For this review, take the finished solid that the model builds, in its own axes (mm). A direction names the side the tool comes from. Coordinates: 2 decimals unless noted, no trailing zeros. Write each loop counter-clockwise with the first axis right and the second up, starting at its lowest first coordinate (ties: lowest second). Pieces come first, ordered by that corner, then holes. Notation, with made-up numbers: (-37, -3.5) - (-13, -3.5) arc R34 cw to (-13, 28.5) - close; hole circle Ø5 at (57.5, 20). An arc over 180 degrees is marked (long way). Use one line per item in the form item = value. Start each with the question number.
1) Mouldability with a two-part tool opening along Z and no side actions: class faces 4 (the flat face through (-12, 0, -1)), 5 (the flat face through (-2, 5, 37)) as pulls with the +Z half, pulls with the -Z half, needs draft (parallel to the pull), parting line crosses it, or undercut.
2) We need section C-C (x = -50). Give the boundary of the cut face in (y, z).
3) We need section D-D (z = 50.5). Give the boundary of the cut face in (x, y), plus the area to 3 significant figures.
4) Tool access review of faces 1 (the cylindrical face through (-34.94, 8.45, 12.73)), 2 (the cylindrical face through (14.898, 2.465, 39.316)), 3 (the cylindrical face through (-5.41, 4.51, 5.34)): name each direction out of +Z, -Z, +X, -X, +Y, -Y from which nothing blocks a thin tool from reaching the whole face with its end or side.
5) We need section B-B (x = -20). Give the boundary of the cut face in (y, z), plus the area to 3 significant figures.
6) For L1, parallel to X at y = 11.75, z = -14; L2, parallel to Z at x = 16, y = 9; L3, parallel to X at y = 6.75, z = 27.5, list the stretches that pass through material, from the lowest coordinate up. Write a range as from..to.
7) We need section A-A (z = -20). Give the boundary of the cut face in (x, y), plus the area to 3 significant figures.
8) Insertion check: P1, Ø12, axis at y = 17, z = -36, coming from the -X side; P2, Ø2, axis at x = -10, y = 4.5, coming from the +Z side; P3, Ø8, axis at x = -17, y = 7.5, coming from the +Z side. Each pin has a flat end and moves straight along its axis. Give the tip position at first contact, or say it passes through.
```python
from build123d import *

# Parameters (mm, degrees)
SKETCH_1_R           = 59
EXTRUDE_1_DEPTH      = 20
SKETCH_2_R           = 44.5
CUT_EXTRUDE_1_DEPTH  = 8
SKETCH_3_R           = 30.1
CUT_EXTRUDE_2_DEPTH  = 6.5
SKETCH_4_R           = 2.1
CUT_EXTRUDE_3_DEPTH  = 86.802097876
SKETCH_5_R           = 3.75
CUT_EXTRUDE_4_DEPTH  = 5
M6X1_0_2_D           = 5
SKETCH_26_R          = 3.1
CUT_EXTRUDE_14_DEPTH = 1.2
CUT_EXTRUDE_17_DEPTH = 2
FILLET_1_R           = 1
SKETCH_29_R          = 1.6
CUT_EXTRUDE_18_DEPTH = 86.530345492


with BuildPart() as part:
    # 草图1 → 凸台-拉伸1 (new body)
    with BuildSketch(Plane(origin=(0, 0, 0), x_dir=(1, 0, 0), z_dir=(0, 1, 0))):
        with Locations(Location((0, 0, 0), (0, 0, 270))):
            Circle(SKETCH_1_R)
    extrude(amount=EXTRUDE_1_DEPTH)

    # 草图2 → 切除-拉伸1 (cut)
    with BuildSketch(Plane(origin=(0, 20, 0), x_dir=(1, 0, 0), z_dir=(0, 1, 0))):
        with Locations(Location((0, 0, 0), (0, 0, 270))):
            Circle(SKETCH_2_R)
    extrude(amount=-CUT_EXTRUDE_1_DEPTH, mode=Mode.SUBTRACT)

    # 草图3 → 切除-拉伸2 (cut)
    with BuildSketch(Plane(origin=(0, 12, 0), x_dir=(1, 0, 0), z_dir=(0, 1, 0))):
        with Locations(Location((0, 0, 0), (0, 0, 270))):
            Circle(SKETCH_3_R)
    extrude(amount=-CUT_EXTRUDE_2_DEPTH, mode=Mode.SUBTRACT)

    # 草图4 → 切除-拉伸3 (cut, through all)
    with BuildSketch(Plane.XZ):
        with Locations(Location((0, 38.5, 0), (0, 0, 270))):
            Circle(SKETCH_4_R)
        with Locations(Location((14.733312146, 35.569362002, 0), (0, 0, 270))):
            Circle(SKETCH_4_R)
        with Locations(Location((27.223611076, 27.223611076, 0), (0, 0, 270))):
            Circle(SKETCH_4_R)
        with Locations(Location((35.569362002, 14.733312146, 0), (0, 0, 270))):
            Circle(SKETCH_4_R)
        with Locations(Location((38.5, 0, 0), (0, 0, 270))):
            Circle(SKETCH_4_R)
        with Locations(Location((35.569362002, -14.733312146, 0), (0, 0, 270))):
            Circle(SKETCH_4_R)
        with Locations(Location((27.223611076, -27.223611076, 0), (0, 0, 270))):
            Circle(SKETCH_4_R)
        with Locations(Location((14.733312146, -35.569362002, 0), (0, 0, 270))):
            Circle(SKETCH_4_R)
        with Locations(Location((0, -38.5, 0), (0, 0, 270))):
            Circle(SKETCH_4_R)
        with Locations(Location((-14.733312146, -35.569362002, 0), (0, 0, 270))):
            Circle(SKETCH_4_R)
        with Locations(Location((-27.223611076, -27.223611076, 0), (0, 0, 270))):
            Circle(SKETCH_4_R)
        with Locations(Location((-35.569362002, -14.733312146, 0), (0, 0, 270))):
            Circle(SKETCH_4_R)
        with Locations(Location((-38.5, 0, 0), (0, 0, 270))):
            Circle(SKETCH_4_R)
        with Locations(Location((-35.569362002, 14.733312146, 0), (0, 0, 270))):
            Circle(SKETCH_4_R)
        with Locations(Location((-27.223611076, 27.223611076, 0), (0, 0, 270))):
            Circle(SKETCH_4_R)
        with Locations(Location((-14.733312146, 35.569362002, 0), (0, 0, 270))):
            Circle(SKETCH_4_R)
    extrude(amount=-CUT_EXTRUDE_3_DEPTH, mode=Mode.SUBTRACT)

    # 草图5 → 切除-拉伸4 (cut)
    with BuildSketch(Plane.XZ):
        with Locations(Location((0, 38.5, 0), (0, 0, 270))):
            Circle(SKETCH_5_R)
        with Locations(Location((14.733312146, 35.569362002, 0), (0, 0, 270))):
            Circle(SKETCH_5_R)
        with Locations(Location((27.223611076, 27.223611076, 0), (0, 0, 270))):
            Circle(SKETCH_5_R)
        with Locations(Location((35.569362002, 14.733312146, 0), (0, 0, 270))):
            Circle(SKETCH_5_R)
        with Locations(Location((38.5, 0, 0), (0, 0, 270))):
            Circle(SKETCH_5_R)
        with Locations(Location((35.569362002, -14.733312146, 0), (0, 0, 270))):
            Circle(SKETCH_5_R)
        with Locations(Location((27.223611076, -27.223611076, 0), (0, 0, 270))):
            Circle(SKETCH_5_R)
        with Locations(Location((14.733312146, -35.569362002, 0), (0, 0, 270))):
            Circle(SKETCH_5_R)
        with Locations(Location((0, -38.5, 0), (0, 0, 270))):
            Circle(SKETCH_5_R)
        with Locations(Location((-14.733312146, -35.569362002, 0), (0, 0, 270))):
            Circle(SKETCH_5_R)
        with Locations(Location((-27.223611076, -27.223611076, 0), (0, 0, 270))):
            Circle(SKETCH_5_R)
        with Locations(Location((-35.569362002, -14.733312146, 0), (0, 0, 270))):
            Circle(SKETCH_5_R)
        with Locations(Location((-38.5, 0, 0), (0, 0, 270))):
            Circle(SKETCH_5_R)
        with Locations(Location((-35.569362002, 14.733312146, 0), (0, 0, 270))):
            Circle(SKETCH_5_R)
        with Locations(Location((-27.223611076, 27.223611076, 0), (0, 0, 270))):
            Circle(SKETCH_5_R)
        with Locations(Location((-14.733312146, 35.569362002, 0), (0, 0, 270))):
            Circle(SKETCH_5_R)
    extrude(amount=-CUT_EXTRUDE_4_DEPTH, mode=Mode.SUBTRACT)

    # M6x1.0 螺纹孔2 (through all)
    with Locations(Plane(origin=(0, 0, 0), x_dir=(-1, 0, 0), z_dir=(0, -1, 0))):
        with Locations((0, 20), (-20, 0), (0, -20), (20, 0)):
            Hole(M6X1_0_2_D / 2)

    # 草图26 → 切除-拉伸14 (cut)
    with BuildSketch(Plane.XZ):
        with Locations(Location((0, 0, 0), (0, 0, 270))):
            Circle(SKETCH_26_R)
    extrude(amount=-CUT_EXTRUDE_14_DEPTH, mode=Mode.SUBTRACT)

    # 草图28 → 切除-拉伸17 (cut)
    with BuildSketch(Plane(origin=(0, 5.5, 0), x_dir=(1, 0, 0), z_dir=(0, 1, 0))):
        with BuildLine():
            Line((-2.1, 11), (-2.1, 7.304108433))
            ThreePointArc((-2.1, 7.304108433), (0, 7.6), (2.1, 7.304108433))
            Line((2.1, 7.304108433), (2.1, 11))
            ThreePointArc((2.1, 11), (0, 13.1), (-2.1, 11))
        make_face()
        with BuildLine():
            ThreePointArc((2.1, 5), (0, 2.9), (-2.1, 5))
            Line((-2.1, 5), (-2.1, 7.304108433))
            ThreePointArc((-2.1, 7.304108433), (-5.374011537, 5.374011537), (-7.304108433, 2.1))
            Line((-7.304108433, 2.1), (-5, 2.1))
            ThreePointArc((-5, 2.1), (-2.9, 0), (-5, -2.1))
            Line((-5, -2.1), (-7.304108433, -2.1))
            ThreePointArc((-7.304108433, -2.1), (-5.374011537, -5.374011537), (-2.1, -7.304108433))
            Line((-2.1, -7.304108433), (-2.1, -5))
            ThreePointArc((-2.1, -5), (0, -2.9), (2.1, -5))
            Line((2.1, -5), (2.1, -7.304108433))
            ThreePointArc((2.1, -7.304108433), (5.374011537, -5.374011537), (7.304108433, -2.1))
            Line((7.304108433, -2.1), (5, -2.1))
            ThreePointArc((5, -2.1), (2.9, 0), (5, 2.1))
            Line((5, 2.1), (7.304108433, 2.1))
            ThreePointArc((7.304108433, 2.1), (5.374011537, 5.374011537), (2.1, 7.304108433))
            Line((2.1, 7.304108433), (2.1, 5))
        make_face()
        with BuildLine():
            ThreePointArc((-7.304108433, -2.1), (-7.6, 0), (-7.304108433, 2.1))
            Line((-7.304108433, 2.1), (-11, 2.1))
            ThreePointArc((-11, 2.1), (-13.1, 0), (-11, -2.1))
            Line((-11, -2.1), (-7.304108433, -2.1))
        make_face()
        with BuildLine():
            ThreePointArc((2.1, -7.304108433), (0, -7.6), (-2.1, -7.304108433))
            Line((-2.1, -7.304108433), (-2.1, -11))
            ThreePointArc((-2.1, -11), (0, -13.1), (2.1, -11))
            Line((2.1, -11), (2.1, -7.304108433))
        make_face()
        with BuildLine():
            Line((11, 2.1), (7.304108433, 2.1))
            ThreePointArc((7.304108433, 2.1), (7.525663562, 1.060371612), (7.6, 0))
            ThreePointArc((7.6, 0), (7.525663562, -1.060371612), (7.304108433, -2.1))
            Line((7.304108433, -2.1), (11, -2.1))
            ThreePointArc((11, -2.1), (13.1, 0), (11, 2.1))
        make_face()
        with BuildLine():
            Line((-2.1, 7.304108433), (-2.1, 5))
            ThreePointArc((-2.1, 5), (0, 2.9), (2.1, 5))
            Line((2.1, 5), (2.1, 7.304108433))
            ThreePointArc((2.1, 7.304108433), (0, 7.6), (-2.1, 7.304108433))
        make_face()
        with BuildLine():
            Line((-5, 2.1), (-7.304108433, 2.1))
            ThreePointArc((-7.304108433, 2.1), (-7.6, 0), (-7.304108433, -2.1))
            Line((-7.304108433, -2.1), (-5, -2.1))
            ThreePointArc((-5, -2.1), (-2.9, 0), (-5, 2.1))
        make_face()
        with BuildLine():
            ThreePointArc((7.6, 0), (7.525663562, 1.060371612), (7.304108433, 2.1))
            Line((7.304108433, 2.1), (5, 2.1))
            ThreePointArc((5, 2.1), (2.9, 0), (5, -2.1))
            Line((5, -2.1), (7.304108433, -2.1))
            ThreePointArc((7.304108433, -2.1), (7.525663562, -1.060371612), (7.6, 0))
        make_face()
        with BuildLine():
            Line((-2.1, -5), (-2.1, -7.304108433))
            ThreePointArc((-2.1, -7.304108433), (0, -7.6), (2.1, -7.304108433))
            Line((2.1, -7.304108433), (2.1, -5))
            ThreePointArc((2.1, -5), (0, -2.9), (-2.1, -5))
        make_face()
    extrude(amount=-CUT_EXTRUDE_17_DEPTH, mode=Mode.SUBTRACT)

    # 圆角1
    fillet_1_edges = [part.edges().sort_by_distance(p)[0] for p in [
        (-7.304108433, 4.5, -2.1),
        (-2.1, 4.5, -7.304108433),
        (2.1, 4.5, -7.304108433),
        (7.304108433, 4.5, -2.1),
        (7.304108433, 4.5, 2.1),
        (2.1, 4.5, 7.304108433),
        (-2.1, 4.5, 7.304108433),
        (-7.304108433, 4.5, 2.1),
    ]]
    fillet(fillet_1_edges, radius=FILLET_1_R)

    # 草图29 → 切除-拉伸18 (cut, through all)
    with BuildSketch(Plane.XZ.offset(-1.2)):
        with Locations(Location((0, 0, 0), (0, 0, 270))):
            Circle(SKETCH_29_R)
    extrude(amount=-CUT_EXTRUDE_18_DEPTH, mode=Mode.SUBTRACT)


solid = part.part
```
Determined:
q1.face_4 = needs draft
q1.face_5 = undercut
q2.outline = (0, -31.32) - (20, -31.32) - (20, 31.32) - (0, 31.32) - close
q3.outline = (-30.51, 0) - (30.51, 0) - (30.51, 20) - (-30.51, 20) - close
q3.area = 1,220 mm²
q4.face_1 = +Y, -Y
q4.face_2 = -Y
q4.face_3 = +Y
q5.outline = (0, -55.51) - (20, -55.51) - (20, -39.75) - (12, -39.75) - (12, -22.49) - (5.5, -22.49) - (5.5, -2.5) - (0, -2.5) - close; (0, 2.5) - (5.5, 2.5) - (5.5, 22.49) - (12, 22.49) - (12, 39.75) - (20, 39.75) - (20, 55.51) - (0, 55.51) - close
q5.area = 1,260 mm²
q6.L1 = -57.31..-37.54, -33.6..-26.65, 26.65..33.6, 37.54..57.31
q6.L2 = -56.79..-37.24, -33.89..-25.5, 25.5..33.89, 37.24..56.79
q6.L3 = -52.2..-29.31, -25.14..-12.24, 12.24..25.14, 29.31..52.2
q7.outline = (-55.51, 0) - (-2.5, 0) - (-2.5, 5.5) - (-22.49, 5.5) - (-22.49, 12) - (-39.75, 12) - (-39.75, 20) - (-55.51, 20) - close; (2.5, 0) - (55.51, 0) - (55.51, 20) - (39.75, 20) - (39.75, 12) - (22.49, 12) - (22.49, 5.5) - (2.5, 5.5) - close
q7.area = 1,260 mm²
q8.P1 = -50.8
q8.P2 = 58.31
q8.P3 = 57.55
